Geometry check sheet. Reference: the model listing, model coordinates, mm. A direction names the side the tool comes from. Round coordinates to 2 decimals unless told otherwise and drop trailing zeros. Order: outer loops, then holes, each group sorted by start corner. A loop starts at its lowest first (then second) coordinate and runs counter-clockwise, first axis right, second up. Notation, with made-up numbers: (81, -25) -> (111, -25) arc R21 ccw to (111, -4) -> close; hole circle Ø6 at (25, 21.5). An arc over 180 degrees is marked (long way). Use a Markdown table: item, result. Add a question column.
Item 1: Sectioned sample at D-D, the plane x = 0.5. Record the cut outline in (y, z), and give its area (3 significant figures).
Item 2: Sectioned sample at C-C, the plane x = -2.25. Record the cut outline in (y, z), and give its area (3 significant figures).
Item 3: Gauge pin test, flat ends, axial feed: pin 1 Ø1 at (x, z) = (-1, 1.5) entering from +Y; pin 2 Ø1.5 at (y, z) = (3, 2) entering from -X; pin 3 Ø1 at (x, y) = (0.5, 2) entering from +Z; pin 4 Ø1.5 at (y, z) = (0.5, 2) entering from +X. Record the tip position at first contact, or that the pin passes through.
Item 4: Material ranges on probe 1 along X at (y, z) = (1.55, 1.85); probe 2 along X at (y, z) = (2, 1.85); probe 3 along Y at (x, z) = (0.75, 1), recorded low to high. Write a range as [from, to].
Item 5: Sectioned sample at B-B, the plane z = 1.45. Record the cut outline in (x, y).
Item 6: Mould release check, pull along X, two halves, no side actions. Record for faces 3 (the cylindrical face through (3.256, 3.626, 1.252)), 4 (the cylindrical face through (0.786, 3.873, 1.252)), 5 (the flat face through (-4.703, 1.412, 1.252)): pulls with the +X half, pulls with the -X half, needs draft (parallel to the pull), parting line crosses it, or undercut.
Item 7: Sectioned sample at A-A, the plane y = 0.4. Record the cut outline in (x, z), and give its area (3 significant figures).
Item 8: Set-up check for faces 1 (the flat face through (4.723, 1.373, 1.252)), 2 (the flat face through (-4.215, 1.249, 1.252)): record each of +Z, -Z, +X, -X, +Y, -Y from which the full face is reachable in a straight line by a thin tool's end or side.
from build123d import *

# Parameters (mm, degrees)
BOSS_EXTRUDE1_DEPTH = 2.54


with BuildPart() as part:
    # Sketch1 → Boss-Extrude1 (new body)
    with BuildSketch(Plane.XY):
        with BuildLine():
            Line((-4.853491174, 0), (-3.559199198, 2.53375457))
            Line((-3.559199198, 2.53375457), (-3.348230277, 2.871336194))
            ThreePointArc((-3.348230277, 2.871336194), (-2.944103246, 3.224381504), (-2.468700609, 3.473283052))
            ThreePointArc((-2.468700609, 3.473283052), (-2.030100497, 3.620676512), (-1.585680864, 3.749463464))
            ThreePointArc((-1.585680864, 3.749463464), (-0.796949472, 3.872230469), (0, 3.917402206))
            ThreePointArc((0, 3.917402206), (0.796949472, 3.872230469), (1.585680864, 3.749463464))
            ThreePointArc((1.585680864, 3.749463464), (2.030100497, 3.620676512), (2.468700609, 3.473283052))
            ThreePointArc((2.468700609, 3.473283052), (2.944103246, 3.224381504), (3.348230277, 2.871336194))
            Line((3.348230277, 2.871336194), (3.559199198, 2.53375457))
            Line((3.559199198, 2.53375457), (4.853491174, 0))
            Line((4.853491174, 0), (5.423931714, 0))
            Line((5.423931714, 0), (4.00161657, 2.78437753))
            Line((4.00161657, 2.78437753), (3.756428721, 3.176714524))
            ThreePointArc((3.756428721, 3.176714524), (3.248333968, 3.631652605), (2.64503979, 3.949717174))
            ThreePointArc((2.64503979, 3.949717174), (2.177010777, 4.106994166), (1.702656867, 4.244018167))
            ThreePointArc((1.702656867, 4.244018167), (0.855815628, 4.376835426), (0, 4.425416473))
            ThreePointArc((0, 4.425416473), (-0.855815628, 4.376835426), (-1.702656867, 4.244018167))
            ThreePointArc((-1.702656867, 4.244018167), (-2.177010777, 4.106994166), (-2.64503979, 3.949717174))
            ThreePointArc((-2.64503979, 3.949717174), (-3.248333968, 3.631652605), (-3.756428721, 3.176714524))
            Line((-3.756428721, 3.176714524), (-4.00161657, 2.78437753))
            Line((-4.00161657, 2.78437753), (-5.423931714, 0))
            Line((-5.423931714, 0), (-4.853491174, 0))
        make_face()
    extrude(amount=BOSS_EXTRUDE1_DEPTH)


solid = part.part
Found:
| question | item | result |
|---|---|---|
| 1 | outline | (3.9, 0) -> (4.41, 0) -> (4.41, 2.54) -> (3.9, 2.54) -> close |
| 1 | area | 1.29 mm2 |
| 2 | outline | (3.55, 0) -> (4.08, 0) -> (4.08, 2.54) -> (3.55, 2.54) -> close |
| 2 | area | 1.36 mm2 |
| 3 | pin 1 | stops at y = 4.41 |
| 3 | pin 2 | stops at x = -4.27 |
| 3 | pin 3 | passes through |
| 3 | pin 4 | stops at x = 5.42 |
| 4 | probe 1 | x = [-4.63, -4.06], [4.06, 4.63] |
| 4 | probe 2 | x = [-4.4, -3.83], [3.83, 4.4] |
| 4 | probe 3 | y = [3.88, 4.39] |
| 5 | outline | (-5.42, 0) -> (-4.85, 0) -> (-3.56, 2.53) -> (-3.35, 2.87) arc R2.28 cw to (-2.47, 3.47) arc R10.98 cw to (-1.59, 3.75) arc R8.17 cw to (0, 3.92) arc R8.17 cw to (1.59, 3.75) arc R10.98 cw to (2.47, 3.47) arc R2.28 cw to (3.35, 2.87) -> (3.56, 2.53) -> (4.85, 0) -> (5.42, 0) -> (4, 2.78) -> (3.76, 3.18) arc R2.79 ccw to (2.65, 3.95) arc R11.49 ccw to (1.7, 4.24) arc R8.67 ccw to (0, 4.43) arc R8.67 ccw to (-1.7, 4.24) arc R11.49 ccw to (-2.65, 3.95) arc R2.79 ccw to (-3.76, 3.18) -> (-4, 2.78) -> close |
| 6 | face 3 | pulls with the +X half |
| 6 | face 4 | undercut |
| 6 | face 5 | pulls with the -X half |
| 7 | outline | (-5.22, 0) -> (-4.65, 0) -> (-4.65, 2.54) -> (-5.22, 2.54) -> close; (4.65, 0) -> (5.22, 0) -> (5.22, 2.54) -> (4.65, 2.54) -> close |
| 7 | area | 2.90 mm2 |
| 8 | face 1 | +Z, -Z, +X, +Y |
| 8 | face 2 | +Z, -Z, -Y |
